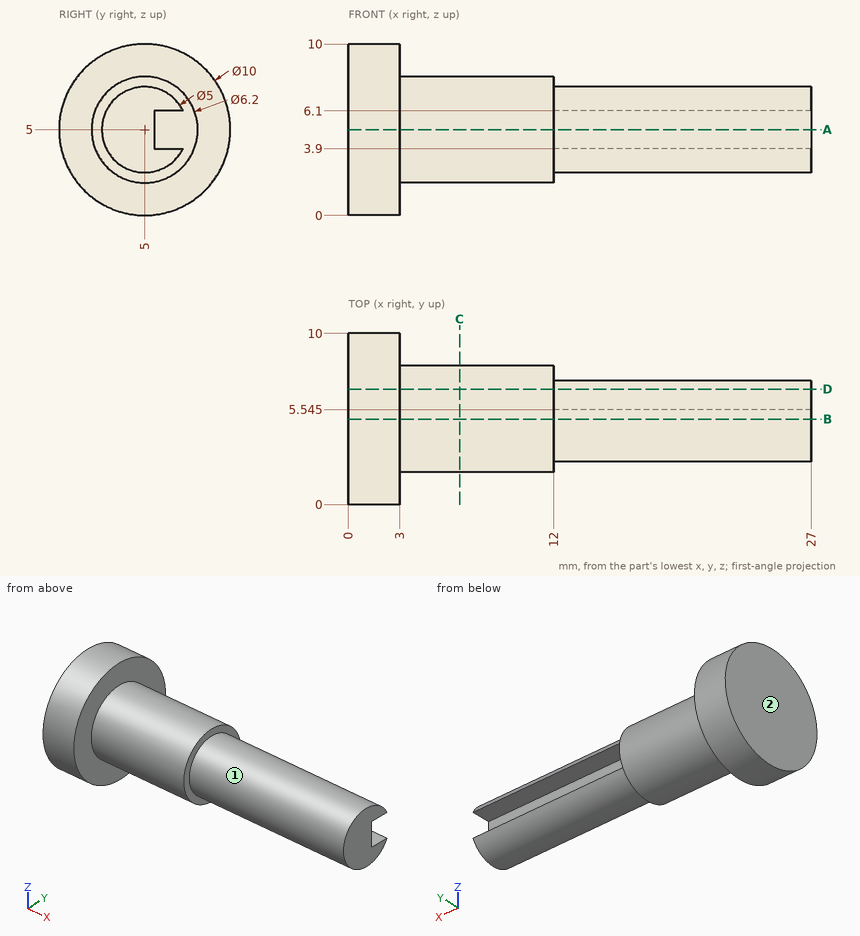
Geometry: see drawing. Coordinates: mm, zero at the bounding-box minimum. A direction names the side the tool comes from. Give positions to 0.01 mm unless a question says otherwise; leave off trailing zeros. Loops run counter-clockwise (first coordinate to the right, second up) from the corner with the lowest first, then second, coordinate; pieces in that order, holes last. Notation, with made-up numbers: (51.5, 86) - (88.5, 86) arc R16 cw to (88.5, 93) - close; hole circle Ø6 at (-7.5, -28). An arc over 180 degrees is marked (long way). Use CSV: the item, a comma, the result in double quotes. Start each with the question number.
1. Section A-A (z = 5). Output: boundary loops of the cut face in (x, y) (3 decimals).
2. Pin query (flat end, axial travel): pin 1 (1.9 mm diameter, centred on x = 18.5, y = 6, fed in from -Z); pin 2 (1.5 mm diameter, centred on x = 4, z = 8, fed in from -Y); pin 3 (0.5 mm diameter, centred on x = 22.5, y = 6.5, fed in from +Z). Return the tip coordinate at first contact, or that it passes through.
3. Ray query, L1, parallel to X at y = 2.5, z = 3.25; L2, parallel to X at y = 1.25, z = 2; L3, parallel to Z at x = 22.25, y = 5.75. Return the intervals inside material, ascending.
4. Section C-C (x = 6.5). Output: boundary loops of the cut face in (y, z).
5. Section B-B (y = 5). Output: boundary loops of the cut face in (x, z), then the cut area to 3 significant figures.
6. Reachability of the marked faces 1 and 2 from +Z, -Z, +X, -X, +Y, -Y: full face, straight path, thin tool, end or side. Return the list, or none.
7. Section D-D (y = 6.75). Output: boundary loops of the cut face in (x, z), then the cut area to 3 significant figures.
Response:
1,outline,"(0, 0) - (3, 0) - (3, 1.9) - (12, 1.9) - (12, 2.5) - (27, 2.5) - (27, 5.545) - (12, 5.545) - (12, 8.1) - (3, 8.1) - (3, 10) - (0, 10) - close"
2,pin 1,"z = 2.5"
2,pin 2,"y = 2.87"
2,pin 3,"z = 7.17"
3,L1,"0 to 12"
3,L2,"0 to 3"
3,L3,"2.62 to 3.9, 6.1 to 7.38"
4,outline,"circle Ø6.2 at (5, 5)"
5,outline,"(0, 0) - (3, 0) - (3, 1.9) - (12, 1.9) - (12, 2.5) - (27, 2.5) - (27, 7.5) - (12, 7.5) - (12, 8.1) - (3, 8.1) - (3, 10) - (0, 10) - close"
5,area,"161 mm²"
6,face 1,"+X"
6,face 2,"+Z, -Z, -X, +Y, -Y"
7,outline,"(0, 0.32) - (3, 0.32) - (3, 2.44) - (12, 2.44) - (12, 3.21) - (27, 3.21) - (27, 3.9) - (12, 3.9) - (12, 6.1) - (27, 6.1) - (27, 6.79) - (12, 6.79) - (12, 7.56) - (3, 7.56) - (3, 9.68) - (0, 9.68) - close"
7,area,"94.7 mm²"
